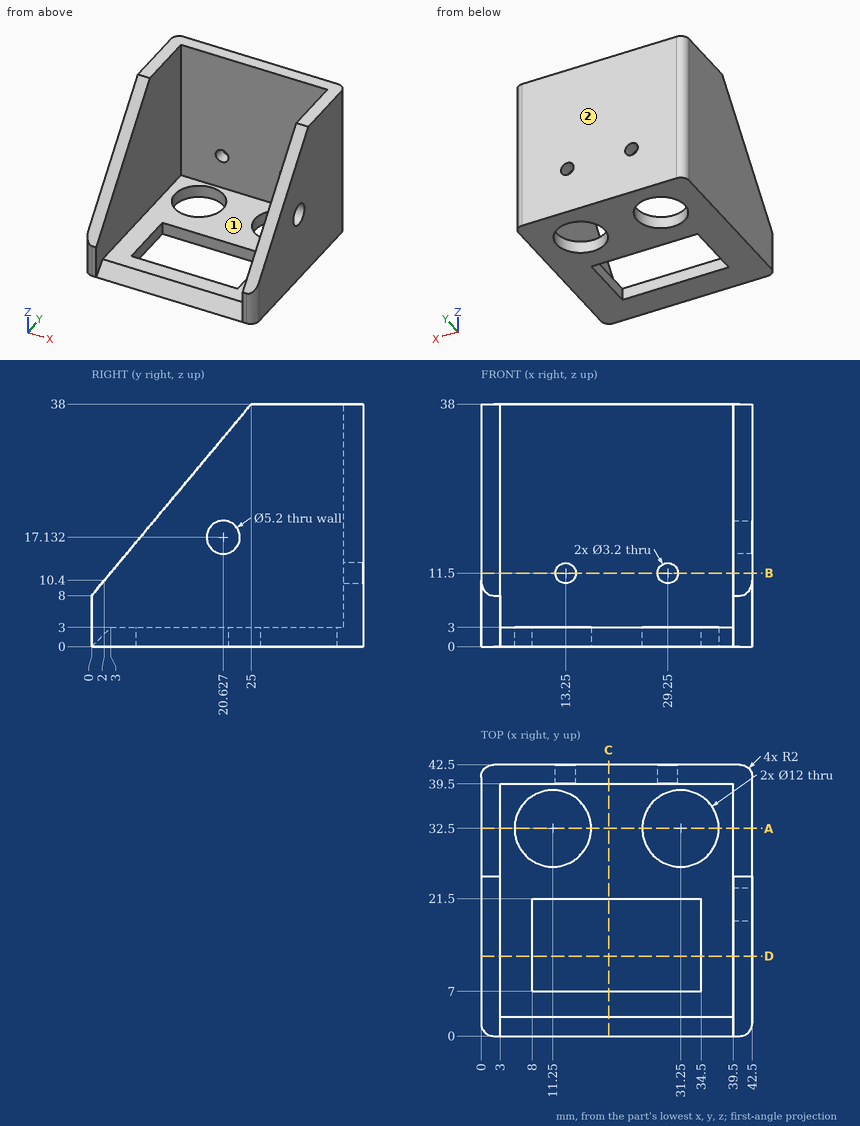
Job drawing, mm, ordinate dimensions from the low corner. One solid piece. A direction names the side the tool comes from. Coordinates: 2 decimals unless noted, no trailing zeros. Write each loop counter-clockwise with the first axis right and the second up, starting at its lowest first coordinate (ties: lowest second). Pieces come first, ordered by that corner, then holes. Notation, with made-up numbers: (50.25, -8) - (70.25, -8) arc R7 ccw to (70.25, 2) - close; hole circle Ø9 at (-22, 30). An arc over 180 degrees is marked (long way). Use a Markdown table: item, result. Add a question column.
Item 1: Flat gauge pins, fed straight in: pin 1 (19 mm diameter, centred on x = 11.25, y = 32.5, fed in from -Z); pin 2 (7 mm diameter, centred on x = 31.25, y = 32.5, fed in from -Z); pin 3 (3.5 mm diameter, centred on x = 13.25, z = 11.5, fed in from -Y); pin 4 (6 mm diameter, centred on x = 33.5, z = 4, fed in from -Y). Where does each tip first touch, or does it go through?
Item 2: Band-saw the part on B-B, the plane z = 11.5. Give the cut face in (x, y).
Item 3: Band-saw the part on C-C, the plane x = 20. Give the cut face in (y, z).
Item 4: Drill centre lines: L1, parallel to X at y = 11, z = 17; L2, parallel to X at y = 32, z = 2; L3, parallel to Y at x = 17, z = 24. Where is each one in solid material? Low to high. Write a range as from..to.
Item 5: Band-saw the part on D-D, the plane y = 12.5. Give the cut face in (x, z), and give its area (3 significant figures).
Item 6: Band-saw the part on A-A, the plane y = 32.5. Give the cut face in (x, z).
Item 7: 3-axis set-ups, long thin cutter, end or side, ignore diameter. For the marked faces 1 and 2: which of +Z, -Z, +X, -X, +Y, -Y reach the whole face in a straight line?
Numbers:
| question | item | result |
|---|---|---|
| 1 | pin 1 | z = 0 |
| 1 | pin 2 | through |
| 1 | pin 3 | y = 39.5 |
| 1 | pin 4 | y = 1 |
| 2 | outline | (0, 2.92) - (3, 2.92) - (3, 39.5) - (11.65, 39.5) - (11.65, 42.5) - (2, 42.5) arc R2 ccw to (0, 40.5) - close; (14.85, 39.5) - (27.65, 39.5) - (27.65, 42.5) - (14.85, 42.5) - close; (30.85, 39.5) - (39.5, 39.5) - (39.5, 2.92) - (42.5, 2.92) - (42.5, 40.5) arc R2 ccw to (40.5, 42.5) - (30.85, 42.5) - close |
| 3 | outline | (0, 0) - (7, 0) - (7, 3) - (3, 3) - close; (21.5, 0) - (42.5, 0) - (42.5, 38) - (39.5, 38) - (39.5, 3) - (21.5, 3) - close |
| 4 | L1 | 0..3, 39.5..42.5 |
| 4 | L2 | 0..5.27, 17.23..25.27, 37.23..42.5 |
| 4 | L3 | 39.5..42.5 |
| 5 | outline | (0, 0) - (8, 0) - (8, 3) - (3, 3) - (3, 23) - (0, 23) - close; (34.5, 0) - (42.5, 0) - (42.5, 23) - (39.5, 23) - (39.5, 3) - (34.5, 3) - close |
| 5 | area | 168 mm2 |
| 6 | outline | (0, 0) - (5.25, 0) - (5.25, 3) - (3, 3) - (3, 38) - (0, 38) - close; (17.25, 0) - (25.25, 0) - (25.25, 3) - (17.25, 3) - close; (37.25, 0) - (42.5, 0) - (42.5, 38) - (39.5, 38) - (39.5, 3) - (37.25, 3) - close |
| 7 | face 1 | +Z, -Y |
| 7 | face 2 | +Z, -Z, +X, -X, +Y |
